Can you work these out from the model? Positions are in its coordinate system, mm. A direction names the side the tool comes from. Round coordinates to 2 decimals unless told otherwise and drop trailing zeros. Loops run counter-clockwise (first coordinate to the right, second up) from the corner with the lowest first, then second, coordinate; pieces in that order, holes last.
```python
from build123d import *

# Parameters (mm, degrees)
SKETCH_R        = 1.45
SKETCH_R_2      = 0.95
PAD_DEPTH       = 5
SKETCH001_R     = 3.562029
SKETCH001_R_2   = 3.731918
SKETCH001_R_3   = 3.520265
SKETCH001_R_4   = 3.380429
POCKET_DEPTH    = 3
SKETCH002_W     = 46.716316
SKETCH002_H     = 3
POCKET001_DEPTH = 3
FILLET_R        = 2
FILLET001_R     = 2
FILLET002_R     = 1
CHAMFER_SIZE    = 1


with BuildPart() as part:
    # Sketch → Pad (new body)
    with BuildSketch(Plane.XY):
        Polygon((-22.586229, 0), (-18.23987, 6.804103), (-18.23987, 16.887657), (-12.328823, 24.143423), (0, 24.143423), (12.328823, 24.143423), (18.23987, 16.887657), (18.23987, 6.804103), (22.586229, 0), (18.23987, -6.804103), (18.23987, -16.887657), (12.328823, -24.148312), (0.02983, -24.148312), (-12.328823, -24.148312), (-18.23987, -16.887657), (-18.23987, -6.804103), align=None)
        with Locations((-15, 15)):
            Circle(SKETCH_R, mode=Mode.SUBTRACT)
        with Locations((0, 17.67767)):
            Circle(SKETCH_R_2, mode=Mode.SUBTRACT)
        with Locations((15, 15)):
            Circle(SKETCH_R, mode=Mode.SUBTRACT)
        with Locations((15, -15)):
            Circle(SKETCH_R, mode=Mode.SUBTRACT)
        with Locations((-15, -15)):
            Circle(SKETCH_R, mode=Mode.SUBTRACT)
        with Locations((0, -17.67767)):
            Circle(SKETCH_R_2, mode=Mode.SUBTRACT)
        with Locations((-17.67767, 0)):
            Circle(SKETCH_R_2, mode=Mode.SUBTRACT)
        with Locations((17.67767, 0)):
            Circle(SKETCH_R_2, mode=Mode.SUBTRACT)
        Polygon((11.207193, -6.470476), (11.207193, 6.470476), (0, 12.940952), (-11.207193, 6.470476), (-11.207193, -6.470476), (0, -12.940952), align=None, mode=Mode.SUBTRACT)
    extrude(amount=PAD_DEPTH)

    # Sketch001 (on Face32 of Pad) → Pocket (cut)
    with BuildSketch(Plane.XY.offset(5)):
        with Locations((-7, -19)):
            Circle(SKETCH001_R)
        with Locations((7, -19)):
            Circle(SKETCH001_R_2)
        with Locations((-7, 19)):
            Circle(SKETCH001_R_3)
        with Locations((7, 19)):
            Circle(SKETCH001_R_4)
    extrude(amount=-POCKET_DEPTH, mode=Mode.SUBTRACT)

    # Sketch002 (on Face5 of Pocket) → Pocket001 (cut)
    with BuildSketch(Plane.XY.offset(5)):
        with Locations((0.200285, -6.541265)):
            Rectangle(SKETCH002_W, SKETCH002_H)
    extrude(amount=-POCKET001_DEPTH, mode=Mode.SUBTRACT)

    # Fillet
    fillet_edges = [part.edges().sort_by_distance(p)[0] for p in [
        (22.586229, 0, 2.5),
        (-22.586229, 0, 2.5),
        (18.23987, -16.887657, 2.5),
        (12.328823, -24.148312, 2.5),
        (-12.328823, -24.148312, 2.5),
        (-18.23987, -16.887657, 2.5),
        (-18.23987, 16.887657, 2.5),
        (-18.23987, 6.804103, 2.5),
        (-18.23987, -6.804103, 1),
        (-12.328823, 24.143423, 2.5),
        (12.328823, 24.143423, 2.5),
        (18.23987, 16.887657, 2.5),
        (18.23987, 6.804103, 2.5),
    ]]
    fillet(fillet_edges, radius=FILLET_R)

    # Fillet001
    fillet001_edges = [part.edges().sort_by_distance(p)[0] for p in [
        (11.207193, -6.470476, 1),
        (0, -12.940952, 2.5),
        (11.207193, 6.470476, 2.5),
        (0, 12.940952, 2.5),
        (-11.207193, 6.470476, 2.5),
        (-11.207193, -6.470476, 1),
    ]]
    fillet(fillet001_edges, radius=FILLET001_R)

    # Fillet002
    fillet002_edges = [part.edges().sort_by_distance(p)[0] for p in [
        (15.286569, -5.041265, 5),
        (13.363188, -8.041265, 5),
        (-15.286569, -5.041265, 5),
        (-13.363188, -8.041265, 5),
    ]]
    fillet(fillet002_edges, radius=FILLET002_R)

    # Chamfer
    chamfer_edges = [part.edges().sort_by_distance(p)[0] for p in [
        (3.619571, 19, 5),
        (-10.520265, 19, 5),
        (3.268082, -19, 5),
        (-10.562029, -19, 5),
    ]]
    chamfer(chamfer_edges, length=CHAMFER_SIZE)


solid = part.part
```
(1) If I drill on line 1 (Y direction, x = 0, z = 3.8); line 2 (Y direction, x = 15, z = 1.55); line 3 (X direction, y = 0.5, z = 2.6), over which ranges is the centre line in solid material (lowest first)?
(2) Suppose I cut it at B-B (x = 0). Write out the boundary of the cut face in (y, z), then the cut area to 3 significant figures.
(3) Suppose I cut it at C-C (x = -15). Write out the boundary of the cut face in (y, z), then the cut area to 3 significant figures.
(4) We'd pull the mould along Y, two halves only. Please class faces 1 (the flat face through (20.501, -3.264, 2.465)), 2 (the cylindrical face through (-12.417, -8.342, 4.715)), 3 (the flat face through (18.24, 12, 2)), 4 (the flat face through (0, 24.143, 2)): released by +Y, released by -Y, zero draft, split by the parting line, or undercut.
(5) Suppose I cut it at A-A (y = 0). Write out the boundary of the cut face in (x, z).
(6) Suppose I cut it at D-D (y = 11). Write out the boundary of the cut face in (x, z).
(7) Which directions (+Z, -Z, +X, -X, +Y, -Y) give clear straight access to the entire face, cutting with the end or side of a thin tool? Please do faces 5 (the flat face through (-14, -7, 2)), 6 (the cylindrical face through (-18.127, -16.838, 2.535)), 7 (the cylindrical face through (6.27, 15.7, 3.01)), 8 (the flat face through (5.668, 9.669, 2.465)).
(8) For pin 1 (4 mm diameter, centred on x = 7, y = 19, fed in from +Z); pin 2 (6 mm diameter, centred on x = 5.5, y = -17.5, fed in from +Z); pin 3 (1 mm diameter, centred on y = 16, z = 1.5, fed in from -X); pin 4 (1 mm diameter, centred on x = -15.5, z = 3, fed in from -Y), each with a flat end and sliding along its axis, tell me the tip position at first contact or that it passes through.
Check result:
1. line 1: y = -24.15 to -18.63, -16.73 to -12.63, 12.63 to 16.73, 18.63 to 24.14
1. line 2: y = -20.87 to -16.45, -13.55 to 13.55, 16.45 to 20.86
1. line 3: x = -22.15 to -18.49, -16.87 to -11.21, 11.21 to 16.87, 18.49 to 22.15
2. outline: (-24.15, 0) - (-18.63, 0) - (-18.63, 5) - (-24.15, 5) - close; (-16.73, 0) - (-12.63, 0) - (-12.63, 5) - (-16.73, 5) - close; (12.63, 0) - (16.73, 0) - (16.73, 5) - (12.63, 5) - close; (18.63, 0) - (24.14, 0) - (24.14, 5) - (18.63, 5) - close
2. area: 96.1 mm2
3. outline: (-20.87, 0) - (-16.45, 0) - (-16.45, 5) - (-20.87, 5) - close; (-13.55, 0) - (13.55, 0) - (13.55, 5) - (-4.04, 5) arc R1 ccw to (-5.04, 4) - (-5.04, 2) - (-8.04, 2) - (-8.04, 4) arc R1 ccw to (-9.04, 5) - (-13.55, 5) - close; (16.45, 0) - (20.86, 0) - (20.86, 5) - (16.45, 5) - close
3. area: 170 mm2
4. face 1: released by -Y
4. face 2: undercut
4. face 3: zero draft
4. face 4: released by +Y
5. outline: (-22.21, 0) - (-18.63, 0) - (-18.63, 5) - (-22.21, 5) - close; (-16.73, 0) - (-11.21, 0) - (-11.21, 5) - (-16.73, 5) - close; (11.21, 0) - (16.73, 0) - (16.73, 5) - (11.21, 5) - close; (18.63, 0) - (22.21, 0) - (22.21, 5) - (18.63, 5) - close
6. outline: (-18.24, 0) - (-3.36, 0) - (-3.36, 5) - (-18.24, 5) - close; (3.36, 0) - (18.24, 0) - (18.24, 5) - (3.36, 5) - close
7. face 5: +Z, +X, -X
7. face 6: +Z, -Z, -X, -Y
7. face 7: +Z
7. face 8: +Z, -Z
8. pin 1: stops at z = 2
8. pin 2: stops at z = 5
8. pin 3: stops at x = -18.24
8. pin 4: stops at y = -20.87
